Model file for the job. Use its own axes, mm. A direction names the side the tool comes from. Round coordinates to 2 decimals unless told otherwise and drop trailing zeros. Use a Markdown table: item, result.
from build123d import *

# Parameters (mm, degrees)
F0_W     = 50
F0_H     = 50
F1_DEPTH = 13
F2_W     = 2
F2_H     = 3
F3_DEPTH = 50.001


with BuildPart() as f1:
    # F0 (on Top) → F1 (new body)
    with BuildSketch(Plane.XY):
        Rectangle(F0_W, F0_H)
    extrude(amount=F1_DEPTH)

    # F2 (on face) → F3 (cut, through all)
    with BuildSketch(Plane(origin=(0, 25, 0), x_dir=(-1, 0, 0), z_dir=(0, 1, 0))):
        with Locations((-20, 11.5)):
            Rectangle(F2_W, F2_H)
        with Locations((-15, 11.5)):
            Rectangle(F2_W, F2_H)
        with Locations((-10, 11.5)):
            Rectangle(F2_W, F2_H)
        with Locations((-5, 11.5)):
            Rectangle(F2_W, F2_H)
        Polygon((1, 13), (-1, 13), (-1, 10), (0, 10), (1, 10), align=None)
        with Locations((5, 11.5)):
            Rectangle(F2_W, F2_H)
        with Locations((10, 11.5)):
            Rectangle(F2_W, F2_H)
        with Locations((15, 11.5)):
            Rectangle(F2_W, F2_H)
        with Locations((20, 11.5)):
            Rectangle(F2_W, F2_H)
    extrude(amount=-F3_DEPTH, mode=Mode.SUBTRACT)


solid = f1.part
Q1. Pull direction X, two halves, no side cores. Call faces 3 (the face through (-25, 0, 6)), 4 (the face through (-13, 0, 13)), 5 (the face through (19, 0, 11)): released by +X, released by -X, zero draft, split by the parting line, or undercut.
Results list:
| item | result |
|---|---|
| face 3 | released by -X |
| face 4 | zero draft |
| face 5 | undercut |
Q2. Drill centre line: L1, parallel to Z at x = 5, y = -11. Where is it in solid material? Low to high. Write a range as from..to.
Results list:
| item | result |
|---|---|
| L1 | z = 0..10 |
Q3. Band-saw the part on A-A, the plane z = 11. Give the number of separate pieces and of enclosed holes in the cut face, plus the area to 3 significant figures.
Results list:
| item | result |
|---|---|
| separate pieces | 10 |
| enclosed holes | 0 |
| area | 1,600 mm² |
Q4. Flat gauge pins, fed straight in: pin 1 (2 mm diameter, centred on x = -5.5, y = -5.5, fed in from +Z); pin 2 (1.6 mm diameter, centred on x = 0, y = -2, fed in from +Z). Where does each tip first touch, or does it go through?
Results list:
| item | result |
|---|---|
| pin 1 | stops at z = 13 |
| pin 2 | stops at z = 10 |
Q5. Tool access for faces 1 (the face through (21, 0, 11)), 2 (the face through (2, 0, 13)): list every direction of +Z, -Z, +X, -X, +Y, -Y with a clear straight run to the whole face (end or side of a thin tool).
Results list:
| item | result |
|---|---|
| face 1 | +Z, +Y, -Y |
| face 2 | +Z, +X, -X, +Y, -Y |
